from build123d import *

# Parameters (mm, degrees)
SKETCH1_W           = 55.1
SKETCH1_H           = 27.8
BOSS_EXTRUDE1_DEPTH = 3
SKETCH3_W           = 21.65
SKETCH3_H           = 20.203759547
SKETCH3_W_2         = 17.65
SKETCH3_H_2         = 15.75
CUT_EXTRUDE1_DEPTH  = 32.00342723
SKETCH4_W           = 19.154601746
SKETCH4_H           = 20.203759547
CUT_EXTRUDE2_DEPTH  = 32.00342723
CUT_EXTRUDE3_DEPTH  = 10
SKETCH7_W           = 4.4
SKETCH7_H           = 3
BOSS_EXTRUDE2_DEPTH = 4.1
SKETCH8_W           = 3.662724417
SKETCH8_H           = 3
SKETCH8_W_2         = 3.933516036
BOSS_EXTRUDE3_DEPTH = 3
SKETCH9_W           = 62.2
SKETCH9_H           = 3
BOSS_EXTRUDE4_DEPTH = 3.21
SKETCH10_W          = 62.2
SKETCH10_H          = 3
BOSS_EXTRUDE5_DEPTH = 3.21
SKETCH12_W          = 34.22
SKETCH12_H          = 3
BOSS_EXTRUDE7_DEPTH = 20
CUT_EXTRUDE4_DEPTH  = 54.451422806
SKETCH14_W          = 2.8
SKETCH14_H          = 2.8
BOSS_EXTRUDE8_DEPTH = 3
SKETCH11_R          = 0.85
BOSS_EXTRUDE9_DEPTH = 3


with BuildPart() as part:
    # Sketch1 → Boss-Extrude1 (new body)
    with BuildSketch(Plane(origin=(0, 0, 0), x_dir=(1, 0, 0), z_dir=(0, 1, 0))):
        Rectangle(SKETCH1_W, SKETCH1_H)
    extrude(amount=BOSS_EXTRUDE1_DEPTH)

    # Sketch3 → Cut-Extrude1 (cut, through all)
    # profile 1 of 2: a face of its own
    with BuildSketch(Plane.XZ):
        with Locations((-12.325, -0.13539581)):
            Rectangle(SKETCH3_W, SKETCH3_H)
        with Locations((-12.325, -0.375)):
            Rectangle(SKETCH3_W_2, SKETCH3_H_2, mode=Mode.SUBTRACT)
    # profile 2 of 2: a face of its own
    with BuildSketch(Plane.XZ):
        with Locations((-12.325, -0.375)):
            Rectangle(SKETCH3_W_2, SKETCH3_H_2)
    extrude(amount=-CUT_EXTRUDE1_DEPTH, mode=Mode.SUBTRACT)

    # Sketch4 → Cut-Extrude2 (cut, through all)
    with BuildSketch(Plane(origin=(0, 3, 0), x_dir=(1, 0, 0), z_dir=(0, 1, 0))):
        with Locations((-32.727300873, 0.13539581)):
            Rectangle(SKETCH4_W, SKETCH4_H)
    extrude(amount=-CUT_EXTRUDE2_DEPTH, mode=Mode.SUBTRACT)

    # Sketch5 → Cut-Extrude3 (cut)
    with BuildSketch(Plane(origin=(0, 3, 0), x_dir=(1, 0, 0), z_dir=(0, 1, 0))):
        Polygon((27.55, -9.5), (27.55, 0), (27.55, 9.5), (21.55, 9.5), (21.55, -9.5), align=None)
    extrude(amount=-CUT_EXTRUDE3_DEPTH, mode=Mode.SUBTRACT)

    # Sketch7 → Boss-Extrude2 (add)
    with BuildSketch(Plane(origin=(27.55, 0, 0), x_dir=(0, 0, -1), z_dir=(1, 0, 0))):
        with Locations((11.7, 1.5)):
            Rectangle(SKETCH7_W, SKETCH7_H)
        with Locations((-11.7, 1.5)):
            Rectangle(SKETCH7_W, SKETCH7_H)
    extrude(amount=BOSS_EXTRUDE2_DEPTH)

    # Sketch8 → Boss-Extrude3 (add)
    with BuildSketch(Plane.ZY.offset(27.55)):
        with Locations((-12.068637792, 1.5)):
            Rectangle(SKETCH8_W, SKETCH8_H)
        with Locations((11.933241982, 1.5)):
            Rectangle(SKETCH8_W_2, SKETCH8_H)
    extrude(amount=BOSS_EXTRUDE3_DEPTH)

    # Sketch9 → Boss-Extrude4 (add)
    with BuildSketch(Plane(origin=(0, 0, -13.9), x_dir=(-1, 0, 0), z_dir=(0, 0, -1))):
        with Locations((-0.55, 1.5)):
            Rectangle(SKETCH9_W, SKETCH9_H)
    extrude(amount=BOSS_EXTRUDE4_DEPTH)

    # Sketch10 → Boss-Extrude5 (add)
    with BuildSketch(Plane.XY.offset(13.9)):
        with Locations((0.55, 1.5)):
            Rectangle(SKETCH10_W, SKETCH10_H)
    extrude(amount=BOSS_EXTRUDE5_DEPTH)

    # Sketch12 → Boss-Extrude7 (add)
    with BuildSketch(Plane.ZY.offset(30.55)):
        with Locations((0, 1.5)):
            Rectangle(SKETCH12_W, SKETCH12_H)
    extrude(amount=BOSS_EXTRUDE7_DEPTH)

    # Sketch13 → Cut-Extrude4 (cut, through all)
    with BuildSketch(Plane(origin=(0, 3, 0), x_dir=(1, 0, 0), z_dir=(0, 1, 0))):
        Polygon((-33.55, 10.237275583), (-33.55, -9.966483964), (-39.942079041, 0.13539581), align=None)
        Polygon((-47.55, 10.237275583), (-47.55, -9.966483964), (-41.157920959, 0.13539581), align=None)
    extrude(amount=-CUT_EXTRUDE4_DEPTH, mode=Mode.SUBTRACT)

    # Sketch14 → Boss-Extrude8 (add)
    with BuildSketch(Plane.XZ):
        with Locations((-47.05, 13.81)):
            Rectangle(SKETCH14_W, SKETCH14_H)
        with Locations((-47.05, -13.81)):
            Rectangle(SKETCH14_W, SKETCH14_H)
        with Locations((-32.05, 13.81)):
            Rectangle(SKETCH14_W, SKETCH14_H)
        with Locations((-32.05, -13.81)):
            Rectangle(SKETCH14_W, SKETCH14_H)
    extrude(amount=BOSS_EXTRUDE8_DEPTH)

    # Sketch11 → Boss-Extrude9 (add)
    with BuildSketch(Plane.XZ):
        with Locations(Location((-16.05, 15.6, 0), (0, 0, 90))):
            Circle(SKETCH11_R)
        with Locations(Location((-16.05, -15.6, 0), (0, 0, 90))):
            Circle(SKETCH11_R)
        with Locations(Location((0.55, -15.6, 0), (0, 0, 90))):
            Circle(SKETCH11_R)
        with Locations(Location((0.55, 15.6, 0), (0, 0, 90))):
            Circle(SKETCH11_R)
        with Locations(Location((17.15, 15.6, 0), (0, 0, 90))):
            Circle(SKETCH11_R)
        with Locations(Location((17.15, -15.6, 0), (0, 0, 90))):
            Circle(SKETCH11_R)
    extrude(amount=BOSS_EXTRUDE9_DEPTH)


solid = part.part
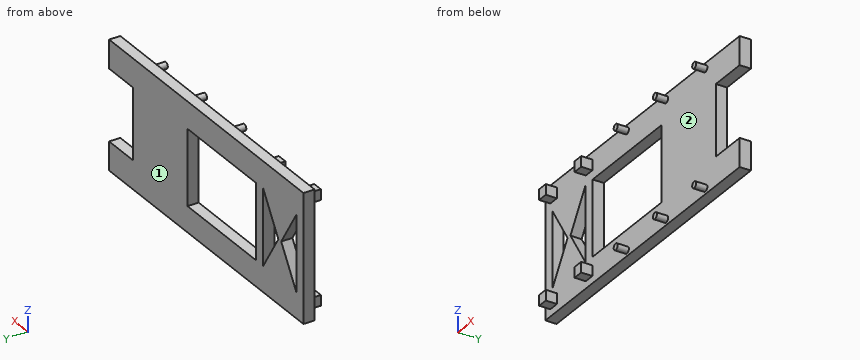
Read the model definition and answer for the solid it produces. Units are mm, in the model's axes. Face numbers are marked on the shaded views. Give positions to 0.01 mm unless a question says otherwise; leave off trailing zeros. Loops run counter-clockwise (first coordinate to the right, second up) from the corner with the lowest first, then second, coordinate; pieces in that order, holes last. Notation, with made-up numbers: (12, -7) -> (33, -7) arc R16 cw to (33, 6) -> close; hole circle Ø8 at (53, 38). An arc over 180 degrees is marked (long way). Answer as CSV lines item,"result".
Item 1: Determine the mould class of the marked faces 1 and 2 for opening direction X: +X half, -X half, draft (parallel to the pull), parting line (faces both ways), or undercut.
Returned:
face 1,"draft"
face 2,"undercut"
Item 2: Each of these flat-tipped pins is pushed along its axis until it touches: pin 1 (1.4 mm diameter, centred on y = -1, z = 13.5, fed in from +X); pin 2 (1.5 mm diameter, centred on y = -2.5, z = 8.5, fed in from -X); pin 3 (2 mm diameter, centred on y = -2, z = -14, fed in from -X); pin 4 (0.8 mm diameter, centred on y = -1, z = -14.5, fed in from +X). Where does it stop, or does it pass through?
Returned:
pin 1,"stops at x = -30.65"
pin 2,"passes through"
pin 3,"stops at x = -48.45"
pin 4,"stops at x = 17.63"
Item 3: Find section B-B on z = -3. Give the vertices of the cut face in (x, y), plus the area to 3 significant figures.
Returned:
outline,"(-50.55, 0) -> (-47.55, 0) -> (-47.55, 3) -> (-50.55, 3) -> close; (-42.97, 0) -> (-38.13, 0) -> (-38.13, 3) -> (-42.97, 3) -> close; (-33.55, 0) -> (-30.55, 0) -> (-30.55, 3) -> (-33.55, 3) -> close; (-1.5, 0) -> (21.55, 0) -> (21.55, 3) -> (-1.5, 3) -> close"
area,"102 mm²"
Item 4: Find section A-A on x = -16.05. Give the vertices of the cut face in (y, z), plus the area to 3 significant figures.
Returned:
outline,"(-3, -16.45) -> (0, -16.45) -> (0, -17.11) -> (3, -17.11) -> (3, -10.24) -> (0, -10.24) -> (0, -14.75) -> (-3, -14.75) -> close; (-3, 14.75) -> (0, 14.75) -> (0, 9.97) -> (3, 9.97) -> (3, 17.11) -> (0, 17.11) -> (0, 16.45) -> (-3, 16.45) -> close"
area,"52.2 mm²"
Item 5: Find section D-D on x = -6. Give the vertices of the cut face in (y, z).
Returned:
outline,"(0, -17.11) -> (3, -17.11) -> (3, -10.24) -> (0, -10.24) -> close; (0, 9.97) -> (3, 9.97) -> (3, 17.11) -> (0, 17.11) -> close"
Item 6: Find section C-C on y = 2. Give the vertices of the cut face in (x, z), plus the area to 3 significant figures.
Returned:
outline,"(-50.55, -17.11) -> (31.65, -17.11) -> (31.65, -9.5) -> (21.55, -9.5) -> (21.55, 9.5) -> (31.65, 9.5) -> (31.65, 17.11) -> (-50.55, 17.11) -> close; hole (-47.55, -10.24) -> (-41.16, -0.14) -> (-47.55, 9.97) -> close; hole (-39.94, -0.14) -> (-33.55, -10.24) -> (-33.55, 9.97) -> close; hole (-30.55, -10.24) -> (-1.5, -10.24) -> (-1.5, 9.97) -> (-30.55, 9.97) -> close"
area,"1,900 mm²"
Item 7: Consider line 1 (Z direction, x = -46.5, y = -1.3); line 2 (Z direction, x = -16, y = 0.1); line 3 (X direction, y = -0.5, z = 15). Determine where each line is inside the solid, lowest interval first. Write a range as [from, to].
Returned:
line 1,"z = [-15.21, -12.41], [12.41, 15.21]"
line 2,"z = [-17.11, -10.24], [9.97, 17.11]"
line 3,"x = [-48.45, -45.65], [-33.45, -30.65], [-16.65, -15.45], [-0.05, 1.15], [16.55, 17.75]"
